Here's how the part is built. I have some questions about the finished solid (model axes, mm). Round coordinates to 2 decimals unless told otherwise and drop trailing zeros. Loops run counter-clockwise (first coordinate to the right, second up) from the corner with the lowest first, then second, coordinate; pieces in that order, holes last. Notation, with made-up numbers: (74.25, 70.25) - (133.25, 70.25) arc R25 cw to (133.25, 102.25) - close; hole circle Ø5 at (-34.5, 69.25). An arc over 180 degrees is marked (long way). Return JSON: item names as keys, results as strings. Group by question number.
```python
from build123d import *

# Parameters (mm, degrees)
SKETCH1_W           = 63.5
SKETCH1_H           = 58.42
BOSS_EXTRUDE1_DEPTH = 15.875
FILLET1_R           = 7.9375


with BuildPart() as part:
    # Sketch1 → Boss-Extrude1 (new body)
    with BuildSketch(Plane(origin=(0, 0, 0), x_dir=(1, 0, 0), z_dir=(0, 1, 0))):
        Rectangle(SKETCH1_W, SKETCH1_H)
    extrude(amount=BOSS_EXTRUDE1_DEPTH)

    # Fillet1
    fillet1_edges = [part.edges().sort_by_distance(p)[0] for p in [
        (0, 15.875, 29.21),
        (0, 15.875, -29.21),
    ]]
    fillet(fillet1_edges, radius=FILLET1_R)


solid = part.part
```
Q1. Will this pin go through, and if not, where does the flat tip stop? pin 1 Ø5 at (x, y) = (-1.5, 14) entering from -Z.
Q2. Imagine slicing it at A-A, the plane x = 25. List the corners of the cut face in (y, z) for me (1 decimal), and give its area (3 significant figures).
Q3. Please list where these lines run through material, in increasing order: line 1 (Y direction, x = 22, z = -27); line 2 (Y direction, x = -24, z = -22); line 3 (Z direction, x = 23, y = 13.5).
Q4. Imagine slicing it at B-B, the plane z = -23.5. List the corners of the cut face in (x, y) for me, and give its area (3 significant figures).
Output values:
{
 "1": {"pin 1": "stops at z = -28.37"},
 "2": {"outline": "(0, -29.2) - (7.9, -29.2) arc R7.9 ccw to (15.9, -21.3) - (15.9, 21.3) arc R7.9 ccw to (7.9, 29.2) - (0, 29.2) - close", "area": "900 mm^2"},
 "3": {"line 1": "y = 0 to 13.43", "line 2": "y = 0 to 15.84", "line 3": "z = -26.93 to 26.93"},
 "4": {"outline": "(-31.75, 0) - (31.75, 0) - (31.75, 15.56) - (-31.75, 15.56) - close", "area": "988 mm^2"}
}
